Here's the drawing with two shaded views (mm, measured from the low corner). I have some questions. A direction names the side the tool comes from. Round coordinates to 2 decimals unless told otherwise and drop trailing zeros. Order: outer loops, then holes, each group sorted by start corner. A loop starts at its lowest first (then second) coordinate and runs counter-clockwise, first axis right, second up.
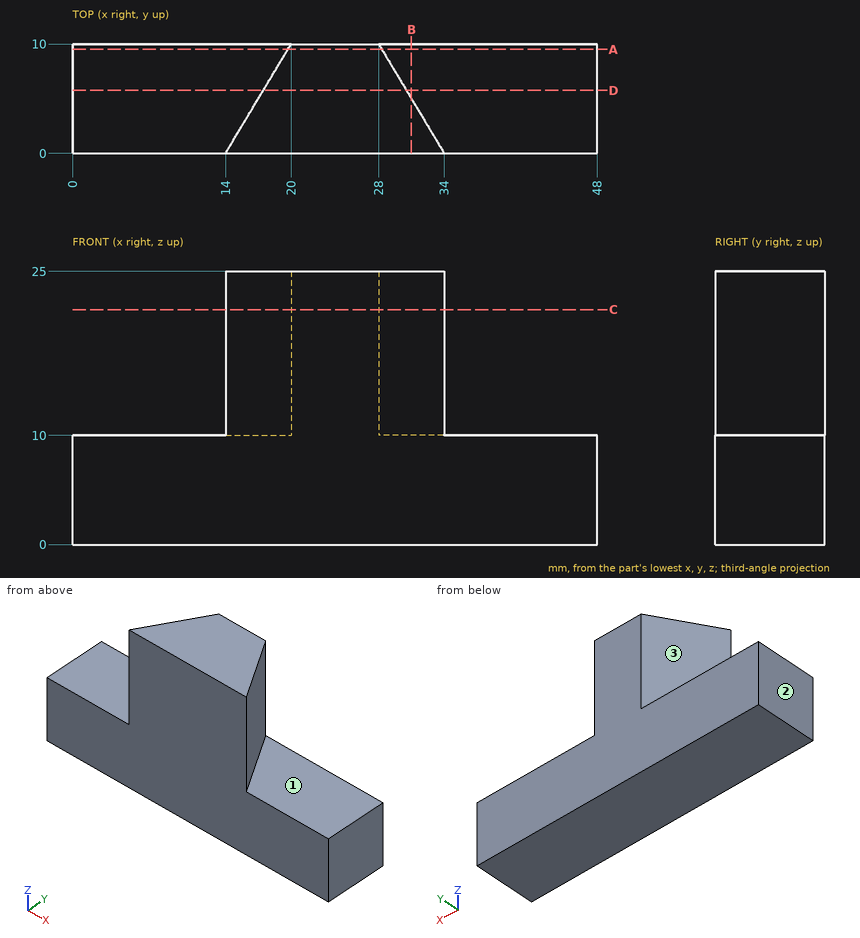
Q1. Imagine slicing it at B-B, the plane x = 31. Please give me the cut outline in (y, z).
Q2. For P1, Ø2, axis at y = 8, z = 22.5, coming from the +X side, with a flat end and sliding along its axis, tell me the tip position at first contact or that it passes through.
Q3. I need wall thicknesses on L1, parallel to Z at x = 41.5, y = 2.75; L2, parallel to X at y = 0.5, z = 11; L3, parallel to X at y = 5.25, z = 19.5. Which ranges of each line are inside material? Lowest first, please.
Q4. Imagine slicing it at D-D, the plane y = 5.75. Please give me the cut outline in (x, z), then the cut area to 4 significant figures.
Q5. For the marked faces 1, 2 and 3, which set-ups out of +Z, -Z, +X, -X, +Y, -Y let a thin tool reach every point of the face, with its end or its side?
Q6. Imagine slicing it at C-C, the plane z = 21.5. Please give me the cut outline in (x, y).
Q7. Imagine slicing it at A-A, the plane y = 9.5. Please give me the cut outline in (x, z).
Filled in:
1. outline: (0, 0) - (10, 0) - (10, 10) - (5, 10) - (5, 25) - (0, 25) - close
2. P1: stops at x = 29.8
3. L1: z = 0 to 10
3. L2: x = 14.3 to 33.7
3. L3: x = 17.15 to 30.85
4. outline: (0, 0) - (48, 0) - (48, 10) - (30.55, 10) - (30.55, 25) - (17.45, 25) - (17.45, 10) - (0, 10) - close
4. area: 676.5 mm2
5. face 1: +Z, +X, +Y
5. face 2: +Z, -Z, -X, +Y, -Y
5. face 3: +Z, -X, +Y
6. outline: (14, 0) - (34, 0) - (28, 10) - (20, 10) - close
7. outline: (0, 0) - (48, 0) - (48, 10) - (28.3, 10) - (28.3, 25) - (19.7, 25) - (19.7, 10) - (0, 10) - close
